from build123d import *

# Parameters (mm, degrees)
BOSS_EXTRUDE1_DEPTH = 7
FILLET1_R           = 3
FILLET2_R           = 5


with BuildPart() as part:
    # Sketch1 → Boss-Extrude1 (new body)
    with BuildSketch(Plane(origin=(0, 0, 0), x_dir=(0, 0, -1), z_dir=(1, 0, 0))):
        Polygon((-21.785617828, -17.377868865), (35.214382172, -17.377868865), (35.214382172, 22.622131135), (23.214382172, 22.622131135), (23.214382172, 16.622131135), (1.187686697, 3.773991719), (3.455005417, -0.113072189), (-20.299274017, -13.968908814), (-22.566592737, -10.081844907), (-42.433808264, -21.670362811), (-38.937098948, -27.665079148), align=None)
        Polygon((23.234116709, 8.569586546), (23.234116709, -10.417868865), (4.764740561, -10.417868865), (4.764740561, -1.399885987), (6.011600394, -1.399885987), align=None, mode=Mode.SUBTRACT)
        Polygon((-39.613886954, -22.304550046), (-34.634489281, -19.42911985), (-33.384302239, -21.59407536), (-38.363699913, -24.469505556), align=None, mode=Mode.SUBTRACT)
        Polygon((-9.735540794, -10.497868865), (-2.235259439, -10.497868865), (-2.235259439, -6.248372162), align=None, mode=Mode.SUBTRACT)
        Polygon((16.699385829, 10.182861543), (17.951839541, 8.019216032), (22.7118599, 10.774614335), (21.459406188, 12.938259845), align=None, mode=Mode.SUBTRACT)
    extrude(amount=-BOSS_EXTRUDE1_DEPTH)

    # Fillet1
    # the kernel refuses this fillet: 3 mm, written as the material it adds along each edge
    with BuildSketch(Plane(origin=(0, -10.417868865, -4.764740561), x_dir=(0, 0, -1), z_dir=(-1, 0, 0))) as fillet1_piece_1:
        with BuildLine():
            CenterArc((FILLET1_R, -FILLET1_R), FILLET1_R, 90, 90)
            Line((0, -FILLET1_R), (-FILLET1_R * 0.02, -FILLET1_R))
            Line((-FILLET1_R * 0.02, -FILLET1_R), (-FILLET1_R * 0.02, FILLET1_R * 0.02))
            Line((-FILLET1_R * 0.02, FILLET1_R * 0.02), (FILLET1_R, FILLET1_R * 0.02))
            Line((FILLET1_R, FILLET1_R * 0.02), (FILLET1_R, 0))
        make_face()
    extrude(amount=7)
    with BuildSketch(Plane(origin=(0, -1.399885987, -4.764740561), x_dir=(0, -1, 0), z_dir=(-1, 0, 0))) as fillet1_piece_2:
        with BuildLine():
            CenterArc((2.434440295, -3), FILLET1_R, 90, 54.240794128)
            Line((0, -1.246859832), (-0.048688806, -1.211797029))
            ThreePointArc((-0.048688806, -1.211797029), (-0.06, -0.623429916), (-0.06, 0))
            Line((-0.06, 0), (0, 0.06))
            Line((0, 0.06), (2.434440295, 0.06))
            Line((2.434440295, 0.06), (2.434440295, 0))
        make_face()
    extrude(amount=7)

    # Fillet2
    fillet2_edges = [part.edges().sort_by_distance(p)[0] for p in [
        (-3.5, -10.417868865, -23.234116709),
    ]]
    fillet(fillet2_edges, radius=FILLET2_R)


solid = part.part
For this review, take the finished solid that the model builds, in its own axes (mm). A direction names the side the tool comes from. Coordinates: 2 decimals unless noted, no trailing zeros. Loops run counter-clockwise (first coordinate to the right, second up) from the corner with the lowest first, then second, coordinate; pieces in that order, holes last. Notation, with made-up numbers: (82, 35) -> (135, 35) arc R7 ccw to (135, 48) -> close; hole circle Ø3 at (3.5, -19.75). An arc over 180 degrees is marked (long way). Write each question's results on one line, items separated by ' | '.
Q1. For pin 1 Ø1.3 at (x, y) = (-5, -8.5) entering from +Z; pin 2 Ø1 at (x, z) = (-1.5, 34) entering from +Y; pin 3 Ø2 at (x, z) = (-3, -12.5) entering from +Y, all flat-tipped, find the tip position at first contact; note any pin that passes through.
Taken from the geometry:
pin 1: z = 12.04 | pin 2: y = -16.46 | pin 3: y = 10.96
Q2. Mouldability with a two-part tool opening along Y and no side actions: class faces 1 (the flat face through (-3.45, 10.29, -12.36)), 2 (the flat face through (-3.451, -20.887, 37.159)), 3 (the flat face through (-3.451, -24.626, 40.71)) as +Y half, -Y half, draft (parallel to the pull), parting line (faces both ways), or undercut.
Taken from the geometry:
face 1: +Y half | face 2: undercut | face 3: -Y half
Q3. To check wall thickness, follow line 1 along Y through (x, z) = (-5.25, -16.5); line 2 along Z through (x, y) = (-5.5, 1.5); line 3 along Z through (x, y) = (-5.5, 4). State the ranges of each line that lie inside material, in increasing order. Write a range as [from, to].
Taken from the geometry:
line 1: [-17.38, -10.42], [4.67, 12.71] | line 2: [-35.21, -23.23], [-11.02, -2.51] | line 3: [-35.21, -23.23], [-15.34, -1.58]
Q4. Machinability: for faces 4 (the flat face through (-3.451, -22.593, 30.481)), 5 (the cylindrical face through (-3.45, -2.48, -5.09)), which of the approach directions +Z, -Z, +X, -X, +Y, -Y give a long, thin tool a straight path to every point of the face, cutting with its end or side? Answer none if there is none.
Taken from the geometry:
face 4: -Z, +X, -X, -Y | face 5: +X, -X
Q5. Add section B-B, the plane y = -3. State the section outline as (x, z) points.
Taken from the geometry:
outline: (-7, -35.21) -> (0, -35.21) -> (0, -23.23) -> (-7, -23.23) -> close; (-7, -4.88) -> (0, -4.88) -> (0, 1.49) -> (-7, 1.49) -> close
Q6. Add section D-D, the plane z = 35.5. State the section outline as (x, y) points, then the cut area to 3 significant figures.
Taken from the geometry:
outline: (-7, -25.6) -> (0, -25.6) -> (0, -22.82) -> (-7, -22.82) -> close; (-7, -19.93) -> (0, -19.93) -> (0, -17.63) -> (-7, -17.63) -> close | area: 35.6 mm²
Q7. Add section A-A, the plane x = -4.25. Count the separate pieces of the cut face and the enclosed holes in it, then the cut area to 3 significant figures.
Taken from the geometry:
separate pieces: 1 | enclosed holes: 4 | area: 1,160 mm²
Q8. Add section C-C, the plane z = -20. State the section outline as (x, y) points, then the cut area to 3 significant figures.
Taken from the geometry:
outline: (-7, -17.38) -> (0, -17.38) -> (0, -10.1) -> (-7, -10.1) -> close; (-7, 6.7) -> (0, 6.7) -> (0, 9.2) -> (-7, 9.2) -> close; (-7, 12.09) -> (0, 12.09) -> (0, 14.75) -> (-7, 14.75) -> close | area: 87.1 mm²
